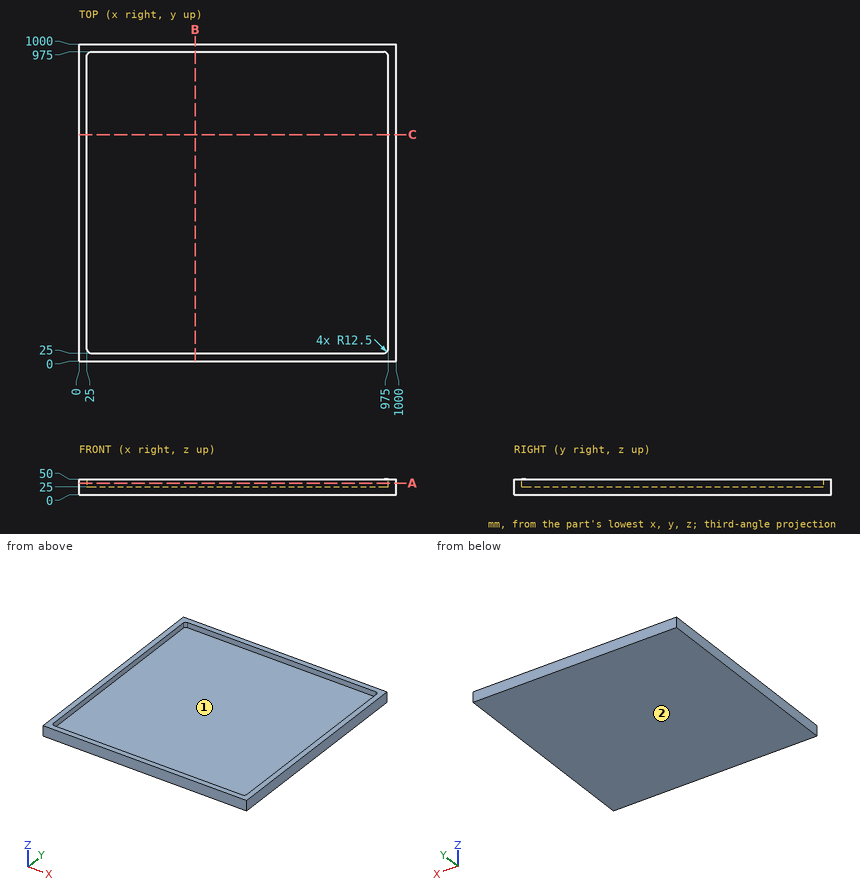
Could you check a few things on this drawing? It's one solid part, dimensions in mm from its lowest x, y, z. Round coordinates to 2 decimals unless told otherwise and drop trailing zeros. Loops run counter-clockwise (first coordinate to the right, second up) from the corner with the lowest first, then second, coordinate; pieces in that order, holes last.
Q1. Please list where these lines run through material, in increasing order: L1, parallel to X at y = 156, z = 44; L2, parallel to Z at x = 481, y = 88.5.
Q2. For P1, Ø3, axis at x = 233, y = 528.5, coming from the +Z side, with a flat end and sliding along its axis, tell me the tip position at first contact or that it passes through.
Q3. I want a section at A-A (z = 37). Write out the boundary of the cut face in (x, y).
Q4. Thinking about a two-plate mould opening in Y: for the marked faces 1 and 2, which applies, pulls with the +Y half, pulls with the -Y half, needs draft (parallel to the pull), parting line crosses it, or undercut?
Q5. I want a section at B-B (x = 366). Write out the boundary of the cut face in (y, z).
Answer below:
1. L1: x = 0 to 25, 975 to 1000
1. L2: z = 0 to 25
2. P1: stops at z = 25
3. outline: (0, 0) - (1000, 0) - (1000, 1000) - (0, 1000) - close; hole (25, 37.5) arc R12.5 ccw to (37.5, 25) - (962.5, 25) arc R12.5 ccw to (975, 37.5) - (975, 962.5) arc R12.5 ccw to (962.5, 975) - (37.5, 975) arc R12.5 ccw to (25, 962.5) - close
4. face 1: undercut
4. face 2: needs draft
5. outline: (0, 0) - (1000, 0) - (1000, 50) - (975, 50) - (975, 25) - (25, 25) - (25, 50) - (0, 50) - close
